For this review, take the finished solid that the model builds, in its own axes (mm). A direction names the side the tool comes from. Round coordinates to 2 decimals unless told otherwise and drop trailing zeros. Order: outer loops, then holes, each group sorted by start corner. A loop starts at its lowest first (then second) coordinate and runs counter-clockwise, first axis right, second up. Notation, with made-up numbers: M -38,86.5 L -24,86.5 A22 ccw -24,99.5 Z; hole C 17,-3.75 d6. An arc over 180 degrees is marked long. Put each result on its own line as item: value.
from build123d import *

# Parameters (mm, degrees)
BOSS_EXTRUDE1_DEPTH = 7.62
CUT_EXTRUDE2_DEPTH  = 6.35
SKETCH7_W           = 1.329001146
SKETCH7_H           = 7.62
BOSS_EXTRUDE2_DEPTH = 12.7
SKETCH8_R           = 3.81
BOSS_EXTRUDE3_DEPTH = 12.7
BOSS_EXTRUDE4_START = 12.7
SKETCH9_R           = 3.81
BOSS_EXTRUDE4_DEPTH = 12.7


with BuildPart() as part:
    # Sketch2 → Boss-Extrude1 (new body)
    with BuildSketch(Plane.XY):
        Polygon((1.329001146, -2.591505287), (1.329001146, 0.714117771), (2.850653855, 0.714117771), (2.850653855, 1.492637762), (1.329001146, 1.492637762), (0, 1.492637762), (0, 0.714117771), (0, -2.591505287), (0, -12.751505287), (1.329001146, -12.751505287), align=None)
    extrude(amount=BOSS_EXTRUDE1_DEPTH)

    # Sketch4 → Cut-Extrude2 (cut)
    with BuildSketch(Plane(origin=(1.329001146, 0, 0), x_dir=(0, 0, -1), z_dir=(1, 0, 0))):
        with BuildLine():
            Line((-3.110701149, -5.332141298), (-3.110701149, -10.010869275))
            ThreePointArc((-3.110701149, -10.010869275), (-3.721619208, -10.928655452), (-4.516161712, -11.693020907))
            Line((-4.516161712, -11.693020907), (-7.62, -11.693020907))
            Line((-7.62, -11.693020907), (-7.62, -2.591505287))
            ThreePointArc((-7.62, -2.591505287), (-4.981588457, -3.330401218), (-3.110701149, -5.332141298))
        make_face()
    extrude(amount=-CUT_EXTRUDE2_DEPTH, mode=Mode.SUBTRACT)

    # Sketch7 → Boss-Extrude2 (add)
    with BuildSketch(Plane.XZ.offset(12.751505287)):
        with Locations((0.664500573, 3.81)):
            Rectangle(SKETCH7_W, SKETCH7_H)
    extrude(amount=BOSS_EXTRUDE2_DEPTH)

    # Sketch8 → Boss-Extrude3 (add)
    with BuildSketch(Plane(origin=(1.329001146, 0, 0), x_dir=(0, 0, -1), z_dir=(1, 0, 0))):
        with Locations((-3.81, -19.101505287)):
            Circle(SKETCH8_R)
    extrude(amount=BOSS_EXTRUDE3_DEPTH)

    # Sketch9 → Boss-Extrude4 (add)
    with BuildSketch(Plane.ZY.offset(BOSS_EXTRUDE4_START)):
        with Locations(Location((3.81, -19.101505287, 0), (0, 0, 180))):
            Circle(SKETCH9_R)
    extrude(amount=-BOSS_EXTRUDE4_DEPTH)


solid = part.part
(1) Draft analysis for pull direction Y (two halves, no side actions). For faces 6 (the face through (1, 1.493, 4)), 7 (the face through (1.329, -6.9, 2.9)), 8 (the face through (0, -6.4, 2.9)), state which applies: released by +Y, released by -Y, zero draft, split by the parting line, or undercut.
A:
face 6: released by +Y
face 7: undercut
face 8: zero draft
(2) To check wall thickness, follow L1, parallel to X at y = -1, z = 4; L2, parallel to Y at x = 1.5, z = 4.25; L3, parallel to Z at x = 2.25, y = -19.25. State the ranges of each line that lie inside material, in increasing order.
A:
L1: x = 0 to 1.33
L2: y = -22.89 to -15.32, 0.71 to 1.49
L3: z = 0 to 7.62
(3) Add section D-D on y = -20.25. Give the boundary of the cut face in (x, z), then the cut area to 3 significant figures.
A:
outline: M -12.7,0.18 L 0,0.18 L 0,0 L 1.33,0 L 1.33,0.18 L 14.03,0.18 L 14.03,7.44 L 1.33,7.44 L 1.33,7.62 L 0,7.62 L 0,7.44 L -12.7,7.44 Z
area: 195 mm2
(4) For faces 1 (the face through (1, -11.693, 6)), 2 (the face through (2, 0.714, 4)), 3 (the face through (0.5, -11.8, 0)), 4 (the face through (7.59, -15.324, 4.306)), 5 (the face through (-6.439, -15.382, 4.636)), list the 3-axis set-ups (+Z, -Z, +X, -X, +Y, -Y) from which the entire face can be reached by the end or side of a thin tool; tool diameter is ignored.
A:
face 1: +Z, +X, -X
face 2: +Z, -Z, +X
face 3: -Z, +X, -X, +Y, -Y
face 4: +X
face 5: -X
(5) Insertion check: pin 1 Ø1.2 at (x, z) = (2.5, 5.5) entering from -Y; pin 2 Ø10 at (x, y) = (3.5, -12.5) entering from +Z; pin 3 Ø4 at (y, z) = (-5.5, 2.5) entering from +X; pin 4 Ø1.5 at (x, z) = (8, 6) entering from -Y. Each pin has a flat end and moves straight along its axis. Give the tip position at first contact, or say it passes through.
A:
pin 1: stops at y = -22.75
pin 2: stops at z = 7.62
pin 3: stops at x = 1.33
pin 4: stops at y = -22.63
(6) Add section C-C on x = -6. Give the boundary of the cut face in (y, z), then the cut area to 3 significant figures.
A:
outline: C -19.1,3.81 d7.62
area: 45.6 mm2
(7) Add section B-B on y = -17.5. Give the boundary of the cut face in (x, z), then the cut area to 3 significant figures.
A:
outline: M -12.7,0.35 L 0,0.35 L 0,0 L 1.33,0 L 1.33,0.35 L 14.03,0.35 L 14.03,7.27 L 1.33,7.27 L 1.33,7.62 L 0,7.62 L 0,7.27 L -12.7,7.27 Z
area: 186 mm2
(8) Add section A-A on z = 5. Give the boundary of the cut face in (x, y), then the cut area to 3 significant figures.
A:
outline: M -12.7,-22.72 L 0,-22.72 L 0,-25.45 L 1.33,-25.45 L 1.33,-22.72 L 14.03,-22.72 L 14.03,-15.48 L 1.33,-15.48 L 1.33,-11.69 L 0,-11.69 L 0,-15.48 L -12.7,-15.48 Z; M 0,-3.32 L 1.33,-3.32 L 1.33,0.71 L 2.85,0.71 L 2.85,1.49 L 0,1.49 Z
area: 210 mm2
